Solid Edge part; units mm, degrees
sketch "Sketch1" plane through (0, 0, 0) normal (0, 0, 1) x (1, 0, 0)
  line L0 (-53.975, -31.75) -> (53.975, -31.75)
  line L1 (53.975, -31.75) -> (53.975, 31.75)
  line L2 (53.975, 31.75) -> (-53.975, 31.75)
  line L3 (-53.975, 31.75) -> (-53.975, -31.75)
  dimension "D1" = 53.975
  dimension "D2" = 53.975
extrude "Protrusion1" add sketch "Sketch1" along normal blind 25.4
chamfer "Chamfer_1" distance 6.35 angle 45 2 edges at (-53.975, 0, 25.4) (53.975, 0, 25.4)
sketch "Sketch2" plane through (53.975, 0, 9.525) normal (1, 0, 0) x (0, 1, 0)
  line L0 (-6.35, 15.875) -> (-31.75, 15.875)
  line L1 (-31.75, 15.875) -> (-31.75, 9.525)
  line L2 (-31.75, 9.525) -> (-6.35, 15.875)
  line L3 (31.75, 15.875) -> (-6.35, 15.875)
  line L4 (-6.35, 15.875) -> (31.75, 9.525)
  line L5 (31.75, 9.525) -> (31.75, 15.875)
extrude "Cutout1" cut sketch "Sketch2" against normal through all
fillet "Round_1" radius 6.35 4 edges at (53.975, -31.75, 9.525) (53.975, 31.75, 9.525) (-53.975, 31.75, 9.525) (-53.975, -31.75, 9.525)
sketch "Sketch3" plane through (-53.975, 0, 9.525) normal (-1, 0, 0) x (0, -1, 0)
  line L0 (-19.05, -3.175) -> (-6.35, -3.175)
  line L1 (-6.35, -3.175) -> (-6.35, 3.175)
  line L2 (-6.35, 3.175) -> (-19.05, 3.175)
  line L3 (-19.05, 3.175) -> (-19.05, -3.175)
  dimension "D1" = 6.35
  dimension "D2" = 6.35
extrude "ExtrudedCutout_3" cut sketch "Sketch3" against normal blind 12.7
sketch "Sketch4" plane through (0, -31.75, 9.525) normal (0, -1, 0) x (1, 0, 0)
  line L0 (-28.575, -3.175) -> (-15.875, -3.175)
  line L1 (-15.875, -3.175) -> (-15.875, 3.175)
  line L2 (-15.875, 3.175) -> (-28.575, 3.175)
  line L3 (-28.575, 3.175) -> (-28.575, -3.175)
  line L4 (-7.9375, -3.175) -> (4.7625, -3.175)
  line L5 (4.7625, -3.175) -> (4.7625, 3.175)
  line L6 (4.7625, 3.175) -> (-7.9375, 3.175)
  line L7 (-7.9375, 3.175) -> (-7.9375, -3.175)
  line L8 (12.7, -3.175) -> (25.4, -3.175)
  line L9 (25.4, -3.175) -> (25.4, 3.175)
  line L10 (25.4, 3.175) -> (12.7, 3.175)
  line L11 (12.7, 3.175) -> (12.7, -3.175)
  line L12 (33.3375, -3.175) -> (46.0375, -3.175)
  line L13 (46.0375, -3.175) -> (46.0375, 3.175)
  line L14 (46.0375, 3.175) -> (33.3375, 3.175)
  line L15 (33.3375, 3.175) -> (33.3375, -3.175)
  dimension "D1" = 15.875
  dimension "D2" = 28.575
extrude "ExtrudedCutout_4" cut sketch "Sketch4" against normal blind 12.7
sketch "Sketch5" plane through (53.975, 0, 9.525) normal (1, 0, 0) x (0, 1, 0)
  circle A0 centre (3.175, 3.175) radius 3.175
  line L0 (11.1125, -3.175) -> (23.8125, -3.175)
  line L1 (23.8125, -3.175) -> (23.8125, 9.525)
  line L2 (23.8125, 9.525) -> (11.1125, 9.525)
  line L3 (11.1125, 9.525) -> (11.1125, -3.175)
extrude "ExtrudedCutout_5" cut sketch "Sketch5" against normal blind 6.35
properties material "ABS Plastic, high impact"
Verification items for the finished model (mm, model axes). A direction names the side the tool comes from. Round coordinates to 2 decimals unless told otherwise and drop trailing zeros. Order: outer loops, then holes, each group sorted by start corner. A loop starts at its lowest first (then second) coordinate and runs counter-clockwise, first axis right, second up. Notation, with made-up numbers: (-37.75, -9.5) - (19.25, -9.5) arc R34 cw to (19.25, 24.5) - close; hole circle Ø2 at (74, 26). An arc over 180 degrees is marked (long way). Use CSV: the item, a comma, the result in double quotes.
(1) Section check A-A on x = 3. Record the boundary of the cut face in (y, z), and give its area (3 significant figures).
Entries:
outline,"(-31.75, 0) - (31.75, 0) - (31.75, 19.05) - (-6.35, 25.4) - (-31.75, 19.05) - (-31.75, 12.7) - (-19.05, 12.7) - (-19.05, 6.35) - (-31.75, 6.35) - close"
area,"1,330 mm^2"
(2) Gauge pin test, flat ends, axial feed: pin 1 Ø1.9 at (y, z) = (14.5, 11) entering from -X (3 decimals); pin 2 Ø1 at (x, y) = (36.5, -15) entering from +Z; pin 3 Ø4 at (x, y) = (-3, -28.5) entering from +Z. Record the tip position at first contact, or that the pin passes through.
Entries:
pin 1,"x = -41.275"
pin 2,"z = 23.36"
pin 3,"z = 20.36"
(3) Thickness scan on probe 1 along X at (y, z) = (-19.5, 11) (1 decimal); probe 2 along X at (y, z) = (21, 11.5) (3 decimals); probe 3 along Z at (x, y) = (20, -27.5). Record the ranges inside material, lowest first. Write a range as from..to.
Entries:
probe 1,"-54..-28.6, -15.9..-7.9, 4.8..12.7, 25.4..33.3, 46..54"
probe 2,"-53.975..47.625"
probe 3,"0..6.35, 12.7..20.11"
(4) Access from +Z, -Z, +X, -X, +Y, -Y to the whole of each face (thin tool, end or side, straight path). Record for faces 4 (the face through (-1, 0, 0)), 5 (the face through (-48, 13, 6.35)), 6 (the face through (1, 31.75, 9)), 7 (the face through (51, 18, 19.05)), 8 (the face through (40, -25, 12.7)).
Entries:
face 4,"-Z, +X, -X, +Y, -Y"
face 5,"-X"
face 6,"+Z, -Z, +X, -X, +Y"
face 7,"+X"
face 8,"-Y"
(5) Mould release check, pull along X, two halves, no side actions. Record for faces 1 (the face through (-22, -25, 6.35)), 2 (the face through (51, 11.112, 13)), 3 (the face through (47.625, 17, 13)): released by +X, released by -X, zero draft, split by the parting line, or undercut.
Entries:
face 1,"undercut"
face 2,"zero draft"
face 3,"released by +X"
